Could you check a few things on this model? Use its own coordinates, in mm. A direction names the side the tool comes from. Give positions to 0.01 mm unless a question says otherwise; leave off trailing zeros. Loops run counter-clockwise (first coordinate to the right, second up) from the corner with the lowest first, then second, coordinate; pieces in that order, holes last. Notation, with made-up numbers: M 6.25,58.25 L 45.25,58.25 A24 cw 45.25,75.25 Z; hole C 44,77.5 d11. An arc over 180 degrees is marked long. Return JSON: item names as keys, results as strings. Group by question number.
1. For faces 1 (the flat face through (8, 0, 0)), 2 (the flat face through (1, 0, 1.01)), which set-ups out of +Z, -Z, +X, -X, +Y, -Y let a thin tool reach every point of the face, with its end or its side?
2. Please list where these lines run through material, in increasing order: line 1 (Z direction, x = 6.75, y = 0.05); line 2 (Y direction, x = 1.25, z = 0.35); line 3 (Y direction, x = 0.5, z = 0.5).
3. For pin 1 (1 mm diameter, centred on x = 2.5, y = -1, fed in from -Z); pin 2 (1 mm diameter, centred on x = 5.5, y = 0.5, fed in from +Z); pin 3 (3 mm diameter, centred on x = 2.5, z = 1.5, fed in from -Y), each with a flat end and sliding along its axis, tell me the tip position at first contact or that it passes through.
4. If we mould it in two halves opening along Z, with no side actions, what happens to faces 3 (the cylindrical face through (4.77, -1.5, 0.07)), 4 (the flat face through (1, 0, -1.01)), 5 (the flat face through (0, 0, -1.2)), 6 (the flat face through (0.592, -0.879, -0.498))? For each: +Z half, -Z half, draft (parallel to the pull), parting line (faces both ways), or undercut.
5. If we section it at B-B (x = 2.75): Write out the boundary of the cut face in (y, z).
6. If we section it at A-A (x = 0.75): Write out the boundary of the cut face in (y, z).
```python
from build123d import *

# Parameters (mm, degrees)
FILLET1_R   = 0.1
HEX_2_DEPTH = 1.2


with BuildPart() as part:
    # BodySke → BaseBody (revolve)
    with BuildSketch(Plane.XY):
        Polygon((0, 0), (0, 2.85), (0.35, 2.85), (1.7, 1.5), (7.7195, 1.5), (8, 1.2195), (8, 0), align=None)
    revolve(axis=Axis((0, 0, 0), (1, 0, 0)))

    # Fillet1
    fillet1_edges = [part.edges().sort_by_distance(p)[0] for p in [
        (1.7, -1.5, 0),
    ]]
    fillet(fillet1_edges, radius=FILLET1_R)

    # Sketch2 → PreBroach (revolve, cut)
    with BuildSketch(Plane.XY):
        Polygon((0, 1.01), (1.2, 1.01), (1.783123772, 0), (0, 0), align=None)
    revolve(axis=Axis((0, 0, 0), (1, 0, 0)), mode=Mode.SUBTRACT)

    # Sketch3 → Hex 2 (cut)
    with BuildSketch(Plane.ZY):
        Polygon((-1.01, -0.583123772), (-1.01, 0.583123772), (0, 1.166247544), (1.01, 0.583123772), (1.01, -0.583123772), (0, -1.166247544), align=None)
    extrude(amount=-HEX_2_DEPTH, mode=Mode.SUBTRACT)


solid = part.part
```
Answer:
{
 "1": {"face 1": "+Z, -Z, +X, +Y, -Y", "face 2": "-X"},
 "2": {"line 1": "z = -1.5 to 1.5", "line 2": "y = -1.92 to -0.85, 0.85 to 1.92", "line 3": "y = -2.65 to -0.88, 0.88 to 2.65"},
 "3": {"pin 1": "stops at z = -1.41", "pin 2": "stops at z = 1.5", "pin 3": "stops at y = -1.87"},
 "4": {"face 3": "parting line", "face 4": "undercut", "face 5": "draft", "face 6": "undercut"},
 "5": {"outline": "C 0,0 d3"},
 "6": {"outline": "C 0,0 d4.9; hole M -1.17,0 L -0.58,-1.01 L 0.58,-1.01 L 1.17,0 L 0.58,1.01 L -0.58,1.01 Z"}
}
